Can you work these out from the model? Positions are in its coordinate system, mm. Round coordinates to 2 decimals unless told otherwise and drop trailing zeros. Order: outer loops, then holes, each group sorted by start corner. A loop starts at its lowest first (then second) coordinate and runs counter-clockwise, first axis right, second up.
Q1. If we section it at A-A (z = -126.5): Please give me the cut outline in (x, y) (1 decimal).
Q2. Will this pin go through, and if not, where does the flat tip stop? P1, Ø4, axis at x = 43.34, z = 206.29, coming from the -Y side.
Q3. If we section it at D-D (y = 1.55): Count the separate pieces of the cut face and the enclosed holes in it, plus the area to 3 significant figures.
Q4. If we section it at B-B (x = 15.5): Please give me the cut outline in (y, z) (3 decimals), plus the area to 3 significant figures.
Q5. If we section it at C-C (x = -65): Please give me the cut outline in (y, z) (3 decimals).
Q6. If I drill on line 1 (X direction, y = 0.85, z = -5); line 2 (X direction, y = 3, z = 192.5); line 3 (Z direction, x = 58.5, y = 1.9), over which ranges is the centre line in solid material (lowest first)?
from build123d import *

# Parameters (mm, degrees)
SKETCH1_W           = 482.6
SKETCH1_H           = 457.2
SKETCH1_R           = 2
SKETCH1_W_2         = 38.1
SKETCH1_H_2         = 12.7
SKETCH1_R_2         = 2.1
SKETCH1_R_3         = 2.0955
SKETCH1_W_3         = 22.197164078
SKETCH1_H_3         = 51.155633978
SKETCH1_H_4         = 36.225516101
SKETCH1_W_4         = 17.438820998
SKETCH1_H_5         = 10.883645004
SKETCH1_W_5         = 19.05
SKETCH1_H_6         = 10.668
BOSS_EXTRUDE1_DEPTH = 3.175
FILLET1_R           = 2.54


with BuildPart() as part:
    # Sketch1 → Boss-Extrude1 (new body)
    with BuildSketch(Plane(origin=(0, 0, 0), x_dir=(1, 0, 0), z_dir=(0, 1, 0))):
        with Locations((-1.251503591, 0)):
            Rectangle(SKETCH1_W, SKETCH1_H)
        with Locations(Location((-172.733503591, -146.082, 0), (0, 0, 270))):
            Circle(SKETCH1_R, mode=Mode.SUBTRACT)
        with Locations((-76.181503591, -186.695610311)):
            Rectangle(SKETCH1_W_2, SKETCH1_H_2, mode=Mode.SUBTRACT)
        with Locations(Location((-39.643603591, -206.2861, 0), (0, 0, 270))):
            Circle(SKETCH1_R_2, mode=Mode.SUBTRACT)
        with BuildLine():
            Line((-166.351503591, -152.4), (-166.351503591, 152.4))
            Line((-166.351503591, 152.4), (138.448496409, 152.4))
            Line((138.448496409, 152.4), (138.448496409, -152.4))
            Line((138.448496409, -152.4), (-140.951503591, -152.4))
            Line((-140.951503591, -152.4), (-140.951503591, -158.75))
            Line((-140.951503591, -158.75), (-158.033759607, -158.75))
            ThreePointArc((-158.033759607, -158.75), (-158.033567596, -158.765999488), (-158.033503591, -158.782))
            ThreePointArc((-158.033503591, -158.782), (-160.049504103, -160.781935995), (-162.033247575, -158.75))
            Line((-162.033247575, -158.75), (-166.351503591, -158.75))
            Line((-166.351503591, -158.75), (-166.351503591, -152.4))
        make_face(mode=Mode.SUBTRACT)
        with Locations(Location((43.338196409, -206.2861, 0), (0, 0, 270))):
            Circle(SKETCH1_R_2, mode=Mode.SUBTRACT)
        with Locations(Location((132.130496409, -158.782, 0), (0, 0, 270))):
            Circle(SKETCH1_R, mode=Mode.SUBTRACT)
        with Locations(Location((144.830496409, -146.082, 0), (0, 0, 270))):
            Circle(SKETCH1_R, mode=Mode.SUBTRACT)
        with Locations(Location((212.390436409, -99.579800078, 0), (0, 0, 270))):
            Circle(SKETCH1_R_3, mode=Mode.SUBTRACT)
        with Locations((194.083935921, -52.428980659)):
            Rectangle(SKETCH1_W_3, SKETCH1_H_3, mode=Mode.SUBTRACT)
        with Locations(Location((-172.733503591, 146.082, 0), (0, 0, 270))):
            Circle(SKETCH1_R, mode=Mode.SUBTRACT)
        with Locations(Location((-160.033503591, 158.782, 0), (0, 0, 270))):
            Circle(SKETCH1_R, mode=Mode.SUBTRACT)
        with Locations(Location((-81.109103591, 184.531, 0), (0, 0, 270))):
            Circle(SKETCH1_R, mode=Mode.SUBTRACT)
        with Locations(Location((-81.109103591, 202.311, 0), (0, 0, 270))):
            Circle(SKETCH1_R, mode=Mode.SUBTRACT)
        with Locations((194.083935921, 4.575109653)):
            Rectangle(SKETCH1_W_3, SKETCH1_H_4, mode=Mode.SUBTRACT)
        with Locations(Location((212.390436409, 89.827999922, 0), (0, 0, 270))):
            Circle(SKETCH1_R_3, mode=Mode.SUBTRACT)
        with Locations((18.318465636, 197.512214728)):
            Rectangle(SKETCH1_W_4, SKETCH1_H_5, mode=Mode.SUBTRACT)
        with Locations(Location((51.351896409, 184.531, 0), (0, 0, 270))):
            Circle(SKETCH1_R, mode=Mode.SUBTRACT)
        with Locations((48.913496409, 193.548)):
            Rectangle(SKETCH1_W_5, SKETCH1_H_6, mode=Mode.SUBTRACT)
        with Locations(Location((51.351896409, 202.311, 0), (0, 0, 270))):
            Circle(SKETCH1_R, mode=Mode.SUBTRACT)
        with Locations(Location((144.830496409, 146.082, 0), (0, 0, 270))):
            Circle(SKETCH1_R, mode=Mode.SUBTRACT)
        with Locations(Location((132.130496409, 158.782, 0), (0, 0, 270))):
            Circle(SKETCH1_R, mode=Mode.SUBTRACT)
    extrude(amount=BOSS_EXTRUDE1_DEPTH)

    # Fillet1
    fillet1_edges = [part.edges().sort_by_distance(p)[0] for p in [
        (-140.951503591, 1.5875, 158.75),
        (-140.951503591, 1.5875, 152.4),
        (-166.351503591, 1.5875, 158.75),
    ]]
    fillet(fillet1_edges, radius=FILLET1_R)


solid = part.part
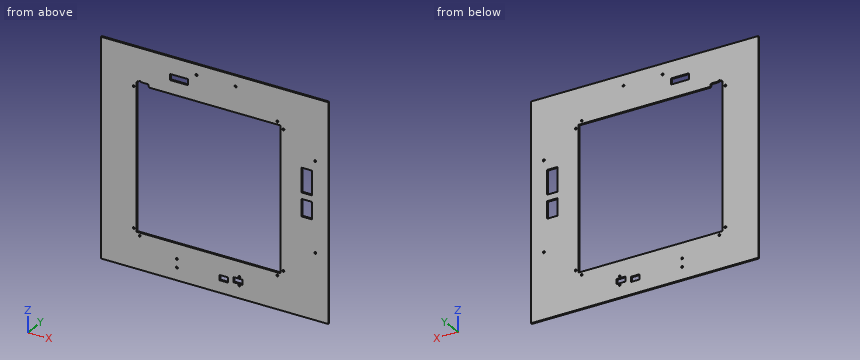
Solution:
1. outline: (-242.6, 0) - (-166.4, 0) - (-166.4, 3.2) - (-242.6, 3.2) - close; (138.4, 0) - (240, 0) - (240, 3.2) - (138.4, 3.2) - close
2. P1: passes through
3. separate pieces: 1
3. enclosed holes: 21
3. area: 125,000 mm2
4. outline: (0, -228.6) - (3.175, -228.6) - (3.175, -202.954) - (0, -202.954) - close; (0, -192.07) - (3.175, -192.07) - (3.175, -152.4) - (0, -152.4) - close; (0, 152.4) - (3.175, 152.4) - (3.175, 228.6) - (0, 228.6) - close
4. area: 449 mm2
5. outline: (0, -228.6) - (3.175, -228.6) - (3.175, -152.4) - (0, -152.4) - close; (0, 152.4) - (3.175, 152.4) - (3.175, 180.346) - (0, 180.346) - close; (0, 193.046) - (3.175, 193.046) - (3.175, 228.6) - (0, 228.6) - close
6. line 1: x = -242.55 to -166.35, 138.45 to 182.99, 205.18 to 240.05
6. line 2: x = -242.55 to -95.23, -57.13 to 240.05
6. line 3: z = -228.6 to -152.4, 152.4 to 228.6
